Source: CAD feature listing. Evaluate the final solid. Frame: model axes, mm. Give positions to 0.01 mm unless a question says otherwise; leave off trailing zeros. Order: outer loops, then holes, each group sorted by start corner. A loop starts at its lowest first (then second) coordinate and runs counter-clockwise, first axis right, second up. Notation, with made-up numbers: (62, 36) - (120, 36) arc R38 ccw to (120, 75) - close; hole circle Ø9 at (-5.75, 4). An arc over 180 degrees is marked (long way). One line per item, written item: value. Start each with the question number.
from build123d import *

# Parameters (mm, degrees)
F0_R     = 100
F2_DEPTH = 10
F3_DEPTH = 10.001
F4_R     = 10
F5_DEPTH = 25
F6_R     = 30
F7_DEPTH = 25


with BuildPart() as f2:
    # F0 (on Front) → F2 (new body)
    with BuildSketch(Plane.XZ):
        Circle(F0_R)
    extrude(amount=F2_DEPTH)

    # F1 (on face) → F3 (cut, through all)
    with BuildSketch(Plane.XZ):
        with BuildLine():
            ThreePointArc((-90, 43.5889894354), (-53.1088554596, 84.7316320613), (0, 100))
            Line((0, 100), (-90, 100))
            Line((-90, 100), (-90, 43.5889894354))
        make_face()
        with BuildLine():
            Line((-90, -43.5889894354), (-90, 43.5889894354))
            ThreePointArc((-90, 43.5889894354), (-100, 0), (-90, -43.5889894354))
        make_face()
        with BuildLine():
            ThreePointArc((100, 0), (97.4679434481, 22.360679775), (90, 43.5889894354))
            Line((90, 43.5889894354), (90, -43.5889894354))
            ThreePointArc((90, -43.5889894354), (97.4679434481, -22.360679775), (100, 0))
        make_face()
    extrude(amount=F3_DEPTH, mode=Mode.SUBTRACT)

    # F4 (on face) → F5 (cut)
    with BuildSketch(Plane.XZ.offset(10)):
        with Locations((-76, 31.4802307404)):
            Circle(F4_R)
        with Locations((-76, -31.4802307404)):
            Circle(F4_R)
        with Locations((-31.4802307404, -76)):
            Circle(F4_R)
        with Locations((31.4802307404, -76)):
            Circle(F4_R)
        with Locations((76, -31.4802307404)):
            Circle(F4_R)
        with Locations((76, 31.4802307404)):
            Circle(F4_R)
        with Locations((31.4802307404, 76)):
            Circle(F4_R)
        with Locations((-31.4802307404, 76)):
            Circle(F4_R)
    extrude(amount=-F5_DEPTH, mode=Mode.SUBTRACT)

    # F6 (on face) → F7 (cut)
    with BuildSketch(Plane.XZ.offset(10)):
        Circle(F6_R)
    extrude(amount=-F7_DEPTH, mode=Mode.SUBTRACT)


solid = f2.part
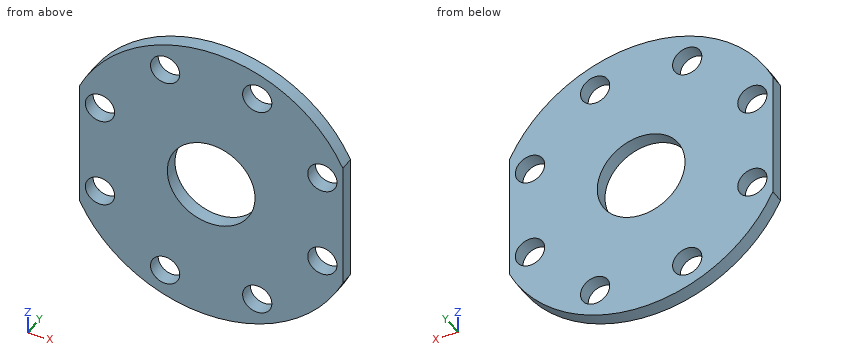
1. Section B-B on x = 0. Return the cut outline in (y, z), then the cut area to 3 significant figures.
2. Section A-A on z = 0. Return the cut outline in (x, y), then the cut area to 3 significant figures.
3. Ray query, L1, parallel to Z at x = 74, y = -5.5; L2, parallel to X at y = -3.25, z = 31; L3, parallel to X at y = -3, z = 68. Return the intervals inside material, ascending.
4. Section C-C on x = -69. Return the cut outline in (y, z), then the cut area to 3 significant figures.
5. Contact query for a flat-ended pin moving along its axis: pin 1 Ø1 at (x, y) = (-28, -8) entering from -Z. Output: stop coordinate, or through.
6. Section D-D on z = -79.5. Return the cut outline in (x, y).
Data:
1. outline: (-10, -100) - (0, -100) - (0, -30) - (-10, -30) - close; (-10, 30) - (0, 30) - (0, 100) - (-10, 100) - close
1. area: 1,400 mm2
2. outline: (-90, -10) - (-30, -10) - (-30, 0) - (-90, 0) - close; (30, -10) - (90, -10) - (90, 0) - (30, 0) - close
2. area: 1,200 mm2
3. L1: z = -67.26 to -41.28, -21.68 to 21.68, 41.28 to 67.26
3. L2: x = -90 to -85.99, -66.01 to 66.01, 85.99 to 90
3. L3: x = -73.32 to -37.48, -25.48 to 25.48, 37.48 to 73.32
4. outline: (-10, -72.38) - (0, -72.38) - (0, -38.62) - (-10, -38.62) - close; (-10, -24.34) - (0, -24.34) - (0, 24.34) - (-10, 24.34) - close; (-10, 38.62) - (0, 38.62) - (0, 72.38) - (-10, 72.38) - close
4. area: 1,160 mm2
5. pin 1: stops at z = -96.14
6. outline: (-60.66, -10) - (-40.85, -10) - (-40.85, 0) - (-60.66, 0) - close; (-22.11, -10) - (22.11, -10) - (22.11, 0) - (-22.11, 0) - close; (40.85, -10) - (60.66, -10) - (60.66, 0) - (40.85, 0) - close
